```python
from build123d import *

# Parameters (mm, degrees)
BOSS_EXTRUDE1_DEPTH = 10
FILLET1_R           = 3
FILLET2_R           = 3
FILLET3_R           = 12
FILLET4_R           = 12
SKETCH2_R           = 5
BOSS_EXTRUDE2_DEPTH = 4
FILLET5_R           = 24


with BuildPart() as part:
    # Sketch1 → Boss-Extrude1 (new body)
    with BuildSketch(Plane(origin=(0, 0, 0), x_dir=(1, 0, 0), z_dir=(0, 1, 0))):
        with BuildLine():
            Line((56, 32), (0, 32))
            Line((0, 32), (0, 0))
            Line((0, 0), (56, 0))
            ThreePointArc((56, 0), (66, -10), (76, 0))
            Line((76, 0), (76, 32))
            ThreePointArc((76, 32), (66, 42), (56, 32))
        make_face()
        with BuildLine():
            ThreePointArc((71, 0), (66, -5), (61, 0))
            ThreePointArc((61, 0), (66, 5), (71, 0))
        make_face(mode=Mode.SUBTRACT)
        with BuildLine():
            ThreePointArc((71, 32), (66, 27), (61, 32))
            ThreePointArc((61, 32), (66, 37), (71, 32))
        make_face(mode=Mode.SUBTRACT)
    extrude(amount=BOSS_EXTRUDE1_DEPTH)

    # Fillet1
    fillet1_edges = [part.edges().sort_by_distance(p)[0] for p in [
        (56, 5, 0),
    ]]
    fillet(fillet1_edges, radius=FILLET1_R)

    # Fillet2
    fillet2_edges = [part.edges().sort_by_distance(p)[0] for p in [
        (56, 5, -32),
    ]]
    fillet(fillet2_edges, radius=FILLET2_R)

    # Fillet3
    fillet3_edges = [part.edges().sort_by_distance(p)[0] for p in [
        (0, 5, -32),
    ]]
    fillet(fillet3_edges, radius=FILLET3_R)

    # Fillet4
    fillet4_edges = [part.edges().sort_by_distance(p)[0] for p in [
        (0, 5, 0),
    ]]
    fillet(fillet4_edges, radius=FILLET4_R)

    # Sketch2 → Boss-Extrude2 (add, symmetric)
    with BuildSketch(Plane.XY.offset(-16)):
        with BuildLine():
            Line((0, 10), (0, 34))
            ThreePointArc((0, 34), (10, 44), (20, 34))
            Line((20, 34), (20, 10))
            Line((20, 10), (0, 10))
        make_face()
        with Locations((10, 34)):
            Circle(SKETCH2_R, mode=Mode.SUBTRACT)
    extrude(amount=BOSS_EXTRUDE2_DEPTH, both=True)

    # Fillet5
    fillet5_edges = [part.edges().sort_by_distance(p)[0] for p in [
        (20, 10, -16),
    ]]
    fillet(fillet5_edges, radius=FILLET5_R - 0.0001)  # a hair under: the kernel refuses the full size


solid = part.part
```
Geometry check sheet. Reference: the model listing, model coordinates, mm. A direction names the side the tool comes from. Round coordinates to 2 decimals unless told otherwise and drop trailing zeros. Write each loop counter-clockwise with the first axis right and the second up, starting at its lowest first coordinate (ties: lowest second). Pieces come first, ordered by that corner, then holes. Notation, with made-up numbers: (-33, -16) -> (5, -16) arc R25 ccw to (5, 9) -> close; hole circle Ø4 at (-9, 53.25). An arc over 180 degrees is marked (long way). Put each result on its own line as item: value.
1) Thickness scan on probe 1 along Z at (x, y) = (66, 5); probe 2 along Y at (x, z) = (10, -15); probe 3 along Z at (x, y) = (17.5, 22). Record the ranges inside material, lowest first. Write a range as from..to.
Recorded:
probe 1: z = -42..-37, -27..-5, 5..10
probe 2: y = 0..29, 39..44
probe 3: z = -20..-12
2) Depth check by flat-ended pin: P1, Ø9, axis at x = 10, y = 34, coming from the +Z side (1 decimal); P2, Ø8, axis at x = 25, y = 5.5, coming from the +Z side; P3, Ø2, axis at y = 35.5, z = -15, coming from the +X side; P4, Ø10, axis at x = 39.5, z = -26, coming from the -Y side. Enter the tip coordinate at first touch or a pass-through.
Recorded:
P1: passes through
P2: stops at z = 0
P3: stops at x = 19.99
P4: stops at y = 0
3) Access from +Z, -Z, +X, -X, +Y, -Y to the whole of each face (thin tool, end or side, straight path). Record for faces 1 (the face through (32, 5, 0)), 2 (the face through (13, 23, -12)), 3 (the face through (13, 23, -20)).
Recorded:
face 1: +Z, -X, +Y, -Y
face 2: +Z, +X, -X, +Y
face 3: -Z, +X, -X, +Y
4) Cross-section at D-D, the plane y = 6. Enter the section's corners in (x, z), plus the area to 3 significant figures.
Recorded:
outline: (0, -20) arc R12 ccw to (12, -32) -> (53.35, -32) arc R3 cw to (56.27, -34.31) arc R10 ccw to (76, -32) -> (76, 0) arc R10 ccw to (56.27, 2.31) arc R3 cw to (53.35, 0) -> (12, 0) arc R12 ccw to (0, -12) -> close; hole circle Ø10 at (66, -32); hole circle Ø10 at (66, 0)
area: 2,530 mm2
5) Cross-section at B-B, the plane y = 31. Enter the section's corners in (x, z).
Recorded:
outline: (0, -20) -> (6, -20) -> (6, -12) -> (0, -12) -> close; (14, -20) -> (20.19, -20) -> (20.19, -12) -> (14, -12) -> close
6) Cross-section at C-C, the plane z = 1. Enter the section's corners in (x, y), plus the area to 3 significant figures.
Recorded:
outline: (55.59, 0) -> (61.1, 0) -> (61.1, 10) -> (55.59, 10) -> close; (70.9, 0) -> (75.95, 0) -> (75.95, 10) -> (70.9, 10) -> close
area: 106 mm2
7) Release check for a two-part mould opening along Z. For faces 4 (the face through (13, 38, -16)), 5 (the face through (33, 5, -32)), 6 (the face through (71, 5, 0)), 7 (the face through (63.693, 4.93, -27.564)) record: pulls with the +Z half, pulls with the -Z half, needs draft (parallel to the pull), parting line crosses it, or undercut.
Recorded:
face 4: needs draft
face 5: pulls with the -Z half
face 6: undercut
face 7: undercut
8) Cross-section at A-A, the plane x = 66. Enter the section's corners in (y, z), plus the area to 3 significant figures.
Recorded:
outline: (0, -42) -> (10, -42) -> (10, -37) -> (0, -37) -> close; (0, -27) -> (10, -27) -> (10, -5) -> (0, -5) -> close; (0, 5) -> (10, 5) -> (10, 10) -> (0, 10) -> close
area: 320 mm2
